Design review of the part built by this model. Coordinates are the model's own, in mm. Face numbers are marked on the shaded views. A direction names the side the tool comes from. Give positions to 0.01 mm unless a question says otherwise; leave off trailing zeros. Loops run counter-clockwise (first coordinate to the right, second up) from the corner with the lowest first, then second, coordinate; pieces in that order, holes last. Notation, with made-up numbers: M 54.25,76.25 L 76.25,76.25 A37 ccw 76.25,113.25 Z; hole C 3,74 d9. An arc over 180 degrees is marked long. Use CSV: the item, a comma, the result in double quotes.
from build123d import *

# Parameters (mm, degrees)
SKETCH1_W           = 127
SKETCH1_H           = 63.5
BOSS_EXTRUDE1_DEPTH = 3
SKETCH2_W           = 3
SKETCH2_H           = 63.5
BOSS_EXTRUDE2_DEPTH = 20
CHAMFER1_SIZE       = 3
SKETCH3_W           = 3
SKETCH3_H           = 10
BOSS_EXTRUDE3_DEPTH = 4


with BuildPart() as part:
    # Sketch1 → Boss-Extrude1 (new body)
    with BuildSketch(Plane(origin=(0, 0, 0), x_dir=(1, 0, 0), z_dir=(0, 1, 0))):
        Rectangle(SKETCH1_W, SKETCH1_H)
    extrude(amount=BOSS_EXTRUDE1_DEPTH)

    # Sketch2 → Boss-Extrude2 (add)
    with BuildSketch(Plane(origin=(0, 3, 0), x_dir=(1, 0, 0), z_dir=(0, 1, 0))):
        with Locations((-62, 0)):
            Rectangle(SKETCH2_W, SKETCH2_H)
        with Locations((62, 0)):
            Rectangle(SKETCH2_W, SKETCH2_H)
    extrude(amount=BOSS_EXTRUDE2_DEPTH)

    # Chamfer1
    chamfer1_edges = [part.edges().sort_by_distance(p)[0] for p in [
        (-60.5, 3, 0),
        (60.5, 3, 0),
    ]]
    chamfer(chamfer1_edges, length=CHAMFER1_SIZE)

    # Sketch3 → Boss-Extrude3 (add)
    with BuildSketch(Plane(origin=(0, 23, 0), x_dir=(1, 0, 0), z_dir=(0, 1, 0))):
        with Locations((-62, 26.75)):
            Rectangle(SKETCH3_W, SKETCH3_H)
        with Locations((-62, -26.75)):
            Rectangle(SKETCH3_W, SKETCH3_H)
        with Locations((62, 26.75)):
            Rectangle(SKETCH3_W, SKETCH3_H)
        with Locations((62, -26.75)):
            Rectangle(SKETCH3_W, SKETCH3_H)
    extrude(amount=BOSS_EXTRUDE3_DEPTH)


solid = part.part
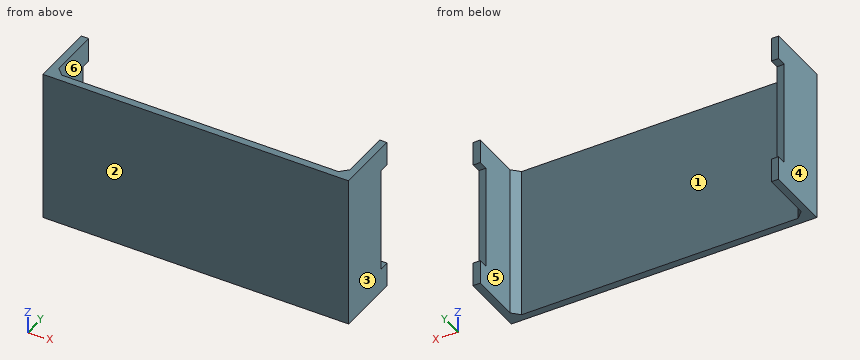
(1) Wall thickness on line 1 along X through (y, z) = (6.25, 6.5); line 2 along Y through (x, z) = (-4, 11); line 3 along X through (y, z) = (4.25, -2): over which ranges is each line inside the solid? List them lowest first. Write a range as [from, to].
A:
line 1,"[-63.5, -60.5], [60.5, 63.5]"
line 2,"[0, 3]"
line 3,"[-63.5, -58.75], [58.75, 63.5]"
(2) We need section B-B on z = -25.5. State the section outline as (x, y) points.
A:
outline,"M -63.5,0 L 63.5,0 L 63.5,27 L 60.5,27 L 60.5,6 L 57.5,3 L -57.5,3 L -60.5,6 L -60.5,27 L -63.5,27 Z"
(3) We need section C-C on x = 42. State the section outline as (y, z) points.
A:
outline,"M 0,-31.75 L 3,-31.75 L 3,31.75 L 0,31.75 Z"
(4) Machinability: for the marked faces 1 and 2, which of the approach directions +Z, -Z, +X, -X, +Y, -Y give a long, thin tool a straight path to every point of the face, cutting with its end or side? Answer none if there is none.
A:
face 1,"+Z, -Z, +Y"
face 2,"+Z, -Z, +X, -X, -Y"
(5) The part is to be moulded in two halves that separate along X. For the marked faces 3, 4, 5 and 6, say which applies: released by +X, released by -X, zero draft, split by the parting line, or undercut.
A:
face 3,"released by +X"
face 4,"released by -X"
face 5,"undercut"
face 6,"undercut"
(6) Clearance check with flat-ended pins moving along their axes: P1, Ø1.5, axis at x = -62.5, z = -5.5, coming from the +Y side; P2, Ø6, axis at x = -35.5, z = 12, coming from the +Y side. State where each tip first meets the part, or that it passes through.
A:
P1,"y = 23"
P2,"y = 3"
(7) We need section D-D on z = -10. State the section outline as (x, y) points.
A:
outline,"M -63.5,0 L 63.5,0 L 63.5,23 L 60.5,23 L 60.5,6 L 57.5,3 L -57.5,3 L -60.5,6 L -60.5,23 L -63.5,23 Z"
(8) We need section A-A on y = 10.25. State the section outline as (x, z) points.
A:
outline,"M -63.5,-31.75 L -60.5,-31.75 L -60.5,31.75 L -63.5,31.75 Z; M 60.5,-31.75 L 63.5,-31.75 L 63.5,31.75 L 60.5,31.75 Z"
